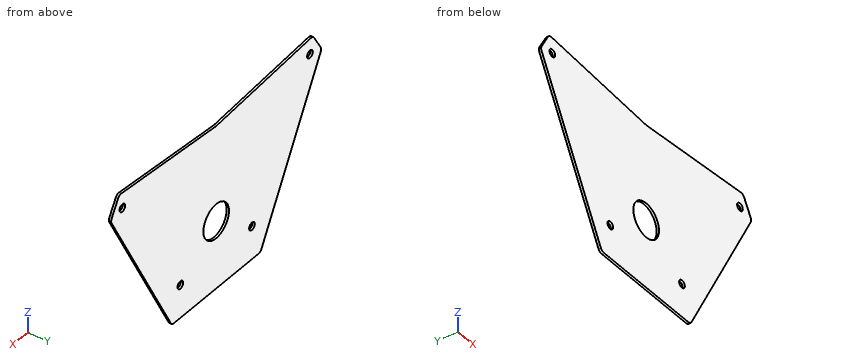
Autodesk Inventor part; units mm, degrees
ref_plane "YZ Plane" through (0, 0, 0) normal (1, 0, 0) x (0, 1, 0)
ref_plane "XZ Plane" through (0, 0, 0) normal (0, 1, 0) x (-1, 0, 0)
ref_plane "XY Plane" through (0, 0, 0) normal (0, 0, 1) x (1, 0, 0)
sketch "Sketch1" plane through (0, 0, 0) normal (0, 1, 0) x (-1, 0, 0)
  line L0 (80.5749, 78.6651) -> (77.2081, 84.4966)
  line L1 (-40.9892, 78.6651) -> (-37.6223, 84.4966)
  line L2 (19.7929, 80.9426) -> (-35.727, 85.4899)
  line L3 (19.7929, 80.9426) -> (75.3128, 85.4899)
  circle A0 centre (-35.159, 78.7632) radius 1.65
  circle A1 centre (74.7448, 78.7632) radius 1.65
  circle A2 centre (-1.1879, 23.9426) radius 1.65
  circle A3 centre (40.7736, 23.9426) radius 1.65
  line L4 (-40.9892, 78.6651) -> (-41.4353, 77.8923)
  line L5 (-41.4699, 75.9547) -> (-6.7517, 10.5409)
  line L6 (-4.9851, 9.4785) -> (44.5709, 9.4785)
  line L7 (80.5749, 78.6651) -> (81.0211, 77.8923)
  line L8 (81.0556, 75.9547) -> (46.3375, 10.5409)
  arc A4 (-35.727, 85.4899) -> (-37.6223, 84.4966) centre (-35.8903, 83.4966) ccw
  arc A5 (77.2081, 84.4966) -> (75.3128, 85.4899) centre (75.476, 83.4966) ccw
  arc A6 (81.0556, 75.9547) -> (81.0211, 77.8923) centre (79.289, 76.8923) ccw
  arc A7 (44.5709, 9.4785) -> (46.3375, 10.5409) centre (44.5709, 11.4785) ccw
  arc A8 (-6.7517, 10.5409) -> (-4.9851, 9.4785) centre (-4.9851, 11.4785) ccw
  arc A9 (-41.4353, 77.8923) -> (-41.4699, 75.9547) centre (-39.7033, 76.8923) ccw
  circle A10 centre (19.7929, 39.09) radius 7.5
extrude "Extrusion1" add sketch "Sketch1" along normal blind 1
properties part number "Verboard Middle Plate" material "Veroboard"
The listing builds one solid part. Answer for the finished solid, in the listing's coordinates (mm). Give positions to 0.01 mm unless a question says otherwise; leave off trailing zeros. Order: outer loops, then holes, each group sorted by start corner. A loop starts at its lowest first (then second) coordinate and runs counter-clockwise, first axis right, second up. Notation, with made-up numbers: (68, 15.5) -> (79, 15.5) arc R25 ccw to (79, 53.5) -> close; hole circle Ø8 at (-24, -23). An arc over 180 degrees is marked (long way). One line per item, written item: value.
1) Find the intervals of material crossed by line 1 (X direction, y = 0.35, z = 22.5); line 2 (Z direction, x = 34.5, y = 0.55); line 3 (Z direction, x = -14, y = 0.7), in increasing order.
Reported:
line 1: x = -52.68 to -41.57, -39.97 to 0.39, 1.99 to 13.1
line 2: z = 62.82 to 77.25, 80.28 to 85.39
line 3: z = 9.48 to 34.33, 43.85 to 81.42
2) Find section B-B, the plane z = 44.5. Determine the outline of the cut face in (x, y).
Reported:
outline: (-64.36, 0) -> (-24.99, 0) -> (-24.99, 1) -> (-64.36, 1) -> close; (-14.6, 0) -> (24.78, 0) -> (24.78, 1) -> (-14.6, 1) -> close
3) Find section D-D, the plane z = 16.5. Determine the outline of the cut face in (x, y), plus the area to 3 significant figures.
Reported:
outline: (-49.5, 0) -> (9.91, 0) -> (9.91, 1) -> (-49.5, 1) -> close
area: 59.4 mm^2
4) Find section C-C, the plane y = 0.7. Determine the outline of the cut face in (x, z), plus the area to 3 significant figures.
Reported:
outline: (-81.06, 75.95) -> (-46.34, 10.54) arc R2 ccw to (-44.57, 9.48) -> (4.99, 9.48) arc R2 ccw to (6.75, 10.54) -> (41.47, 75.95) arc R2 ccw to (41.44, 77.89) -> (40.99, 78.67) -> (37.62, 84.5) arc R2 ccw to (35.73, 85.49) -> (-19.79, 80.94) -> (-75.31, 85.49) arc R2 ccw to (-77.21, 84.5) -> (-80.57, 78.67) -> (-81.02, 77.89) arc R2 ccw to start; hole circle Ø3.3 at (-74.74, 78.76); hole circle Ø3.3 at (-40.77, 23.94); hole circle Ø15 at (-19.79, 39.09); hole circle Ø3.3 at (1.19, 23.94); hole circle Ø3.3 at (35.16, 78.76)
area: 6,470 mm^2
5) Find section A-A, the plane x = -14. Determine the outline of the cut face in (y, z).
Reported:
outline: (0, 9.48) -> (1, 9.48) -> (1, 34.33) -> (0, 34.33) -> close; (0, 43.85) -> (1, 43.85) -> (1, 81.42) -> (0, 81.42) -> close
